Could you check a few things on this model? Use its own coordinates, in mm. A direction names the side the tool comes from. Give positions to 0.01 mm unless a question says otherwise; leave off trailing zeros. Write each loop counter-clockwise with the first axis right and the second up, starting at its lowest first coordinate (ties: lowest second). Pieces come first, ordered by that corner, then holes. Notation, with made-up numbers: (0, 69) - (31, 69) arc R19 ccw to (31, 90) - close; hole circle Ø3 at (-17.75, 62.25). An arc over 180 degrees is marked (long way). Answer as CSV lines item,"result". Start each with the question number.
Q1. On a 3-axis mill with a long thin cutter (end or side, diameter ignored), from which of +Z, -Z, +X, -X, +Y, -Y can I reach the whole of each face in a straight line? I mean faces 1 (the face through (-2.44, 5.25, -0.54)), 2 (the face through (41, 2, 4.5)), 3 (the face through (15.4, 2.5, 3.5)). Say none if no direction works.
Q2. Imagine slicing it at D-D on z = 5.5. List the corners of the cut face in (x, y) for me.
Q3. Imagine slicing it at A-A on z = 0. List the corners of the cut face in (x, y) for me, and give its area (3 significant figures).
Q4. Imagine slicing it at C-C on y = 4.35. List the corners of the cut face in (x, z) for me, and give its area (3 significant figures).
Q5. Will these pins go through, and if not, where does the flat tip stop? pin 1 Ø2 at (x, z) = (36, -6.5) entering from -Y; pin 2 Ø8.5 at (x, z) = (23, -5) entering from +Y; pin 3 Ø1.5 at (x, y) = (12.5, 4) entering from +Z; pin 4 Ø2.5 at (y, z) = (3, -6.5) entering from +X.
Q6. If I drill on line 1 along X through (y, z) = (1.4, 0); line 2 along X through (y, z) = (4.05, 0.5); line 3 along Y through (x, z) = (19, -1.25), over which ranges is the centre line in solid material (lowest first)?
Q7. Imagine slicing it at B-B on x = 31. List the corners of the cut face in (y, z) for me.
Q8. We'd pull the mould along X, two halves only. Please class faces 4 (the face through (41.5, 2, 6)), 5 (the face through (-5.5, 2, -2)), 6 (the face through (18, 0, -2)), 7 (the face through (32.01, 2.71, -1.11)): pulls with the +X half, pulls with the -X half, needs draft (parallel to the pull), parting line crosses it, or undercut.
```python
from build123d import *

# Parameters (mm, degrees)
SKETCH1_R           = 1.5
BOSS_EXTRUDE1_DEPTH = 5
SKETCH2_R           = 2.5
SKETCH2_R_2         = 1.5
BOSS_EXTRUDE2_DEPTH = 0.5


with BuildPart() as part:
    # Sketch1 → Boss-Extrude1 (new body)
    with BuildSketch(Plane(origin=(0, 0, 0), x_dir=(1, 0, 0), z_dir=(0, 1, 0))):
        with BuildLine():
            Line((40.5, -6.5), (41.5, -6.5))
            Line((41.5, -6.5), (41.5, -4.5))
            Line((41.5, -4.5), (40.5, -4.5))
            Line((40.5, -4.5), (40.5, 10.5))
            Line((40.5, 10.5), (-5.5, 10.5))
            Line((-5.5, 10.5), (-5.5, -6.5))
            Line((-5.5, -6.5), (7.562746067, -6.5))
            ThreePointArc((7.562746067, -6.5), (15.5, -3.5), (23.437253933, -6.5))
            Line((23.437253933, -6.5), (40.5, -6.5))
        make_face()
        with Locations(Location((0, 0, 0), (0, 0, 270))):
            Circle(SKETCH1_R, mode=Mode.SUBTRACT)
        with Locations(Location((31, 0, 0), (0, 0, 270))):
            Circle(SKETCH1_R, mode=Mode.SUBTRACT)
    extrude(amount=BOSS_EXTRUDE1_DEPTH)

    # Sketch2 → Boss-Extrude2 (add)
    # profile 1 of 2: a face of its own
    with BuildSketch(Plane(origin=(0, 5, 0), x_dir=(1, 0, 0), z_dir=(0, 1, 0))):
        with Locations(Location((0, 0, 0), (0, 0, 270))):
            Circle(SKETCH2_R)
        with Locations(Location((0, 0, 0), (0, 0, 270))):
            Circle(SKETCH2_R_2, mode=Mode.SUBTRACT)
    # profile 2 of 2: a face of its own
    with BuildSketch(Plane(origin=(0, 5, 0), x_dir=(1, 0, 0), z_dir=(0, 1, 0))):
        with Locations(Location((31, 0, 0), (0, 0, 270))):
            Circle(SKETCH2_R)
        with Locations(Location((31, 0, 0), (0, 0, 270))):
            Circle(SKETCH2_R_2, mode=Mode.SUBTRACT)
    extrude(amount=BOSS_EXTRUDE2_DEPTH)


solid = part.part
```
Conclusion:
1,face 1,"+Y"
1,face 2,"-Z, +X, +Y, -Y"
1,face 3,"+Z, +Y, -Y"
2,outline,"(-5.5, 0) - (8.87, 0) - (8.87, 5) - (-5.5, 5) - close; (22.13, 0) - (41.5, 0) - (41.5, 5) - (22.13, 5) - close"
3,outline,"(-5.5, 0) - (-1.5, 0) - (-1.5, 5.5) - (-2.5, 5.5) - (-2.5, 5) - (-5.5, 5) - close; (1.5, 0) - (29.5, 0) - (29.5, 5.5) - (28.5, 5.5) - (28.5, 5) - (2.5, 5) - (2.5, 5.5) - (1.5, 5.5) - close; (32.5, 0) - (40.5, 0) - (40.5, 5) - (33.5, 5) - (33.5, 5.5) - (32.5, 5.5) - close"
3,area,"202 mm^2"
4,outline,"(-5.5, -10.5) - (40.5, -10.5) - (40.5, 4.5) - (41.5, 4.5) - (41.5, 6.5) - (23.44, 6.5) arc R12 cw to (7.56, 6.5) - (-5.5, 6.5) - close; hole circle Ø3 at (0, 0); hole circle Ø3 at (31, 0)"
4,area,"737 mm^2"
5,pin 1,"y = 0"
5,pin 2,"y = 5"
5,pin 3,"z = 4.1"
5,pin 4,"x = 40.5"
6,line 1,"-5.5 to -1.5, 1.5 to 29.5, 32.5 to 40.5"
6,line 2,"-5.5 to -1.41, 1.41 to 29.59, 32.41 to 40.5"
6,line 3,"0 to 5"
7,outline,"(0, -10.5) - (5, -10.5) - (5, -2.5) - (5.5, -2.5) - (5.5, -1.5) - (0, -1.5) - close; (0, 1.5) - (5.5, 1.5) - (5.5, 2.5) - (5, 2.5) - (5, 6.5) - (0, 6.5) - close"
8,face 4,"pulls with the +X half"
8,face 5,"pulls with the -X half"
8,face 6,"needs draft"
8,face 7,"undercut"
